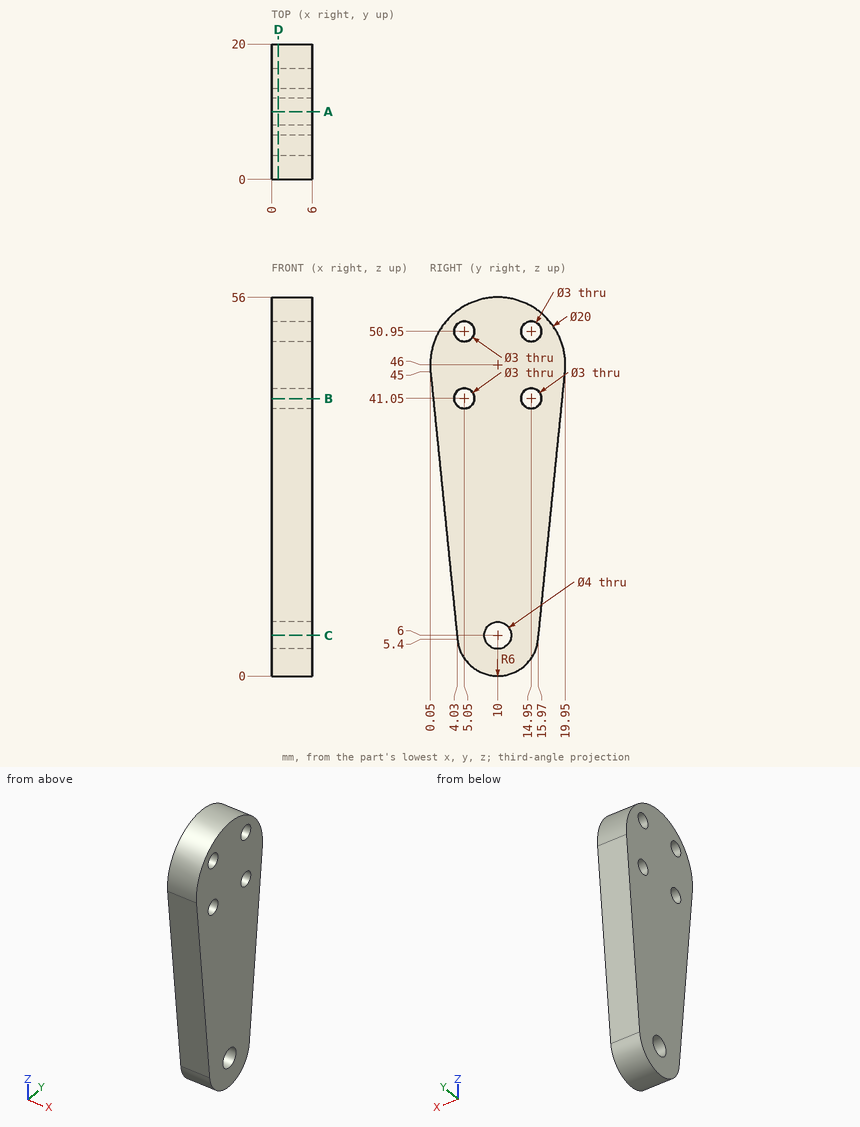
Drawing for the job (mm, zero at the part's lowest x, y, z). Give positions to 0.01 mm unless a question says otherwise; leave off trailing zeros. Loops run counter-clockwise (first coordinate to the right, second up) from the corner with the lowest first, then second, coordinate; pieces in that order, holes last.
Item 1: Slice it at B-B (z = 41). Write the cut outline in (x, y), plus the area to 3 significant figures.
Check values:
outline: (0, 0.45) - (6, 0.45) - (6, 3.55) - (0, 3.55) - close; (0, 6.55) - (6, 6.55) - (6, 13.45) - (0, 13.45) - close; (0, 16.45) - (6, 16.45) - (6, 19.55) - (0, 19.55) - close
area: 78.6 mm2
Item 2: Drop flat-ended pins along their axis: P1, Ø2.5, axis at y = 5.05, z = 50.95, coming from the -X side; P2, Ø5, axis at y = 14.95, z = 41.05, coming from the +X side; P3, Ø2, axis at x = 2, y = 12, coming from the -Z side. Give the stop position or say it passes through.
Check values:
P1: passes through
P2: stops at x = 6
P3: stops at z = 0.08
Item 3: Slice it at C-C (z = 6). Write the cut outline in (x, y).
Check values:
outline: (0, 3.97) - (6, 3.97) - (6, 8) - (0, 8) - close; (0, 12) - (6, 12) - (6, 16.03) - (0, 16.03) - close
Item 4: Slice it at D-D (x = 1). Write the cut outline in (y, z), plus the area to 3 significant figures.
Check values:
outline: (0.05, 45) - (4.03, 5.4) arc R6 ccw to (15.97, 5.4) - (19.95, 45) arc R10 ccw (long way) to start; hole circle Ø3 at (5.05, 41.05); hole circle Ø3 at (5.05, 50.95); hole circle Ø4 at (10, 6); hole circle Ø3 at (14.95, 41.05); hole circle Ø3 at (14.95, 50.95)
area: 816 mm2
Item 5: Slice it at A-A (y = 10). Write the cut outline in (x, z), plus the area to 3 significant figures.
Check values:
outline: (0, 0) - (6, 0) - (6, 4) - (0, 4) - close; (0, 8) - (6, 8) - (6, 56) - (0, 56) - close
area: 312 mm2
Item 6: Drill centre lines: line 1 along Z through (x, y) = (4.75, 14.5); line 2 along Z through (x, y) = (1.5, 6) (1 decimal); line 3 along Z through (x, y) = (2.5, 11.5). Where is each one in solid material? Low to high.
Check values:
line 1: z = 2.03 to 39.62, 42.48 to 49.52, 52.38 to 54.93
line 2: z = 1.5 to 39.9, 42.2 to 49.8, 52.1 to 55.2
line 3: z = 0.19 to 4.68, 7.32 to 55.89
